Study the drawing (mm; zero at the part's minimum x, y, z) and answer. Round coordinates to 2 decimals unless told otherwise and drop trailing zeros. Loops run counter-clockwise (first coordinate to the right, second up) from the corner with the lowest first, then second, coordinate; pieces in that order, holes last. Notation, with made-up numbers: M 88.25,82.5 L 100.25,82.5 A11 cw 100.25,91.5 Z; hole C 35,18 d1. An arc over 180 degrees is marked long. Put each result on its own line as item: value. Start each with the question number.
(1) Section A-A, the plane x = 12.7 is taken. Determine the outline of the cut face in (y, z), then the cut area to 3 significant figures.
(2) Flat-ended cylindrical pins translate along their axes: P1, Ø3, axis at x = 18, z = 19.5, coming from the +Y side; P2, Ø4, axis at x = 6.5, y = 18.5, coming from the +Z side; P3, Ø3, axis at y = 11, z = 15, coming from the +X side; P4, Ø1.5, axis at x = 16, z = 4.5, coming from the +Y side. Find the tip coordinate at first contact, or state that the pin passes through.
(3) Section C-C, the plane z = 13 is taken. Determine the outline of the cut face in (x, y), then the cut area to 3 significant figures.
(4) Straight lines are drawn through the part: line 1 (Y direction, x = 12.7, z = 15.25); line 2 (Z direction, x = 20, y = 14); line 3 (Y direction, x = 6, z = 10.25). For each, find the intervals that lie inside material, in ascending order.
(5) Determine the mould class of the marked faces 1, 2 and 3 for opening direction X: released by +X, released by -X, zero draft, split by the parting line, or undercut.
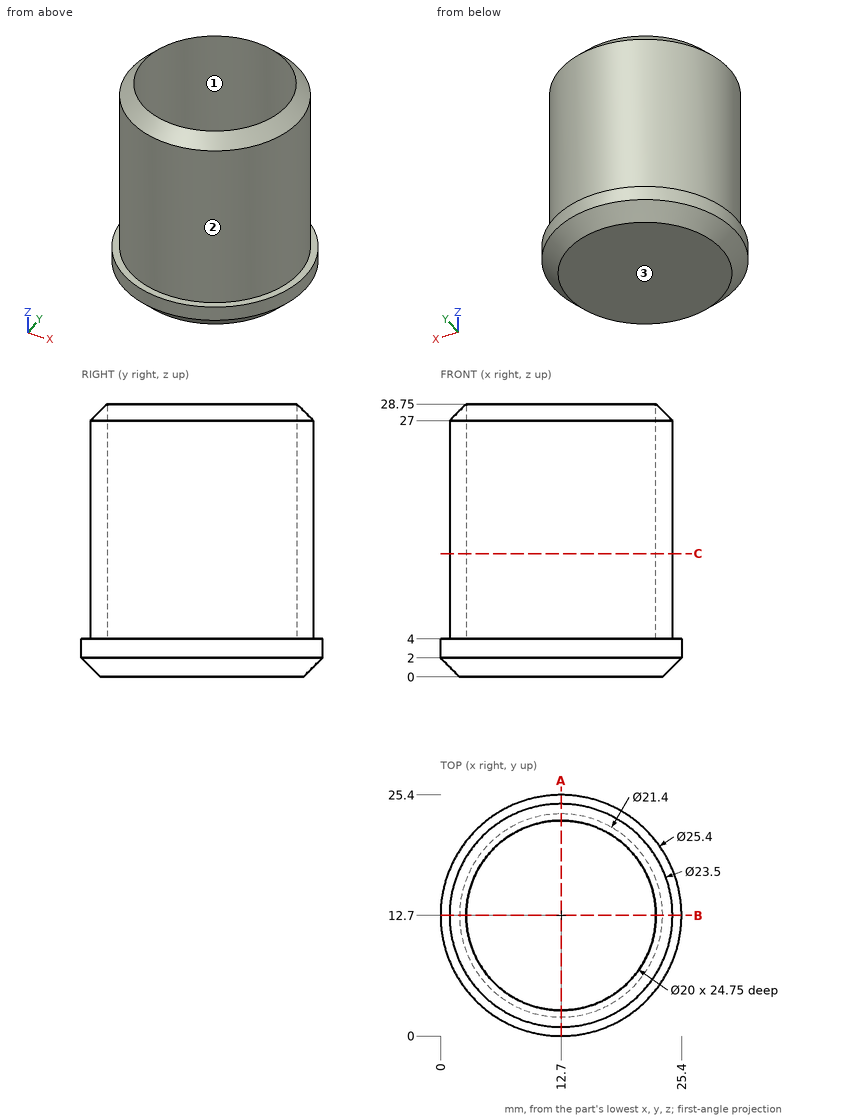
Recorded:
1. outline: M 0,2 L 2,0 L 23.4,0 L 25.4,2 L 25.4,4 L 24.45,4 L 24.45,27 L 22.7,28.75 L 22.7,4 L 2.7,4 L 2.7,28.75 L 0.95,27 L 0.95,4 L 0,4 Z
1. area: 181 mm²
2. P1: stops at y = 23.82
2. P2: stops at z = 28.75
2. P3: stops at x = 24.45
2. P4: stops at y = 25.1
3. outline: C 12.7,12.7 d23.5; hole C 12.7,12.7 d20
3. area: 120 mm²
4. line 1: y = 0.95 to 2.7, 22.7 to 24.45
4. line 2: z = 0 to 4
4. line 3: y = 3.05 to 5.28, 20.12 to 22.35
5. face 1: undercut
5. face 2: split by the parting line
5. face 3: zero draft
